from build123d import *

# Parameters (mm, degrees)
EXTRUDE_1_DEPTH     = 5
SKETCH_2_R          = 2
CUT_EXTRUDE_1_DEPTH = 5


with BuildPart() as part:
    # 草图1 → 凸台-拉伸1 (new body)
    with BuildSketch(Plane.XY):
        with BuildLine():
            ThreePointArc((20, 0), (14.142135624, 14.142135624), (0, 20))
            Line((0, 20), (0, 4.5))
            ThreePointArc((0, 4.5), (3.181980515, 3.181980515), (4.5, 0))
            ThreePointArc((4.5, 0), (3.181980515, -3.181980515), (0, -4.5))
            Line((0, -4.5), (0, -20))
            ThreePointArc((0, -20), (14.142135624, -14.142135624), (20, 0))
        make_face()
        with BuildLine():
            Line((0, 4.5), (0, 20))
            ThreePointArc((0, 20), (-20, 0), (0, -20))
            Line((0, -20), (0, -4.5))
            ThreePointArc((0, -4.5), (-4.5, 0), (0, 4.5))
        make_face()
        with BuildLine():
            Line((70, 20), (0, 20))
            ThreePointArc((0, 20), (14.142135624, 14.142135624), (20, 0))
            ThreePointArc((20, 0), (14.142135624, -14.142135624), (0, -20))
            Line((0, -20), (18.19327595, -28.969251351))
            ThreePointArc((18.19327595, -28.969251351), (20.344914528, -29.738904289), (22.615100256, -30))
            Line((22.615100256, -30), (70, -30))
            Line((70, -30), (70, -27))
            ThreePointArc((70, -27), (68, -25), (70, -23))
            Line((70, -23), (70, -7))
            ThreePointArc((70, -7), (68, -5), (70, -3))
            Line((70, -3), (70, 13))
            ThreePointArc((70, 13), (68, 15), (70, 17))
            Line((70, 17), (70, 20))
        make_face()
        with BuildLine():
            Line((140, 20), (70, 20))
            Line((70, 20), (70, 17))
            ThreePointArc((70, 17), (71.414213562, 16.414213562), (72, 15))
            ThreePointArc((72, 15), (71.414213562, 13.585786438), (70, 13))
            Line((70, 13), (70, -3))
            ThreePointArc((70, -3), (71.414213562, -3.585786438), (72, -5))
            ThreePointArc((72, -5), (71.414213562, -6.414213562), (70, -7))
            Line((70, -7), (70, -23))
            ThreePointArc((70, -23), (71.414213562, -23.585786438), (72, -25))
            ThreePointArc((72, -25), (71.414213562, -26.414213562), (70, -27))
            Line((70, -27), (70, -30))
            Line((70, -30), (117.384899744, -30))
            ThreePointArc((117.384899744, -30), (119.655085472, -29.738904289), (121.80672405, -28.969251351))
            Line((121.80672405, -28.969251351), (140, -20))
            ThreePointArc((140, -20), (120, 0), (140, 20))
        make_face()
        with BuildLine():
            ThreePointArc((160, 0), (154.142135624, 14.142135624), (140, 20))
            Line((140, 20), (140, 4.5))
            ThreePointArc((140, 4.5), (143.181980515, 3.181980515), (144.5, 0))
            ThreePointArc((144.5, 0), (143.181980515, -3.181980515), (140, -4.5))
            Line((140, -4.5), (140, -20))
            ThreePointArc((140, -20), (154.142135624, -14.142135624), (160, 0))
        make_face()
        with BuildLine():
            Line((140, 4.5), (140, 20))
            ThreePointArc((140, 20), (120, 0), (140, -20))
            Line((140, -20), (140, -4.5))
            ThreePointArc((140, -4.5), (135.5, 0), (140, 4.5))
        make_face()
    extrude(amount=EXTRUDE_1_DEPTH)

    # 草图2 → 切除-拉伸1 (cut)
    with BuildSketch(Plane.XY.offset(5)):
        with Locations((22.615100256, -26)):
            Circle(SKETCH_2_R)
        with Locations((117.384899744, -26)):
            Circle(SKETCH_2_R)
    extrude(amount=-CUT_EXTRUDE_1_DEPTH, mode=Mode.SUBTRACT)


solid = part.part
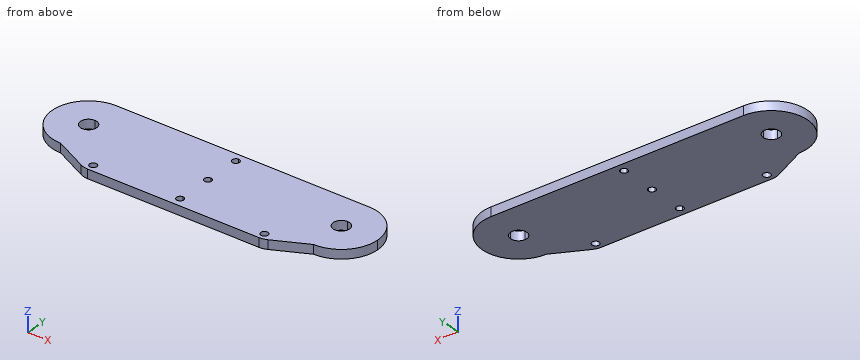
Verification items for the finished model (mm, model axes). Give positions to 0.01 mm unless a question says otherwise; leave off trailing zeros. Write each loop counter-clockwise with the first axis right and the second up, starting at its lowest first coordinate (ties: lowest second). Pieces come first, ordered by that corner, then holes. Notation, with made-up numbers: M 14,-23.75 L 67,-23.75 A25 ccw 67,2.25 Z; hole C 6,-22 d7. An arc over 180 degrees is marked long. Put each result on its own line as item: value. Start each with the question number.
1. Section check C-C (x = 8). Record the cut outline in (y, z).
2. Section check A-A (z = 4.2). Record the cut outline in (x, y), and give its area (3 significant figures).
3. Go/stop test with a flat-tipped pin: pin 1 Ø3.5 at (x, y) = (117.38, -26) entering from -Z. Record where the tip stops, or that it passes through.
4. Scan lines: line 1 along Y through (x, z) = (23.5, 4.75); line 2 along Y through (x, z) = (11, 2.5); line 3 along Y through (x, z) = (132, 1.4). Record each from-to range of solid material in increasing order. Write a range as [from, to].
5. Section check B-B (y = -11). Record the cut outline in (x, z), and give its area (3 significant figures).
Answer list:
1. outline: M -23.94,0 L 20,0 L 20,5 L -23.94,5 Z
2. outline: M 0,-20 L 18.19,-28.97 A10 ccw 22.62,-30 L 117.38,-30 A10 ccw 121.81,-28.97 L 140,-20 A20 ccw 140,20 L 0,20 A20 ccw Z; hole C 0,0 d9; hole C 22.62,-26 d4; hole C 70,-25 d4; hole C 70,-5 d4; hole C 70,15 d4; hole C 117.38,-26 d4; hole C 140,0 d9
2. area: 7,860 mm2
3. pin 1: through
4. line 1: [-30, -27.79], [-24.21, 20]
4. line 2: [-25.42, 20]
4. line 3: [-23.94, 20]
5. outline: M -16.7,0 L 156.7,0 L 156.7,5 L -16.7,5 Z
5. area: 867 mm2
